```python
from build123d import *

# Parameters (mm, degrees)
SKETCH1_W                                = 75
SKETCH1_H                                = 80
BOSS_EXTRUDE1_DEPTH                      = 5
CUT_EXTRUDE1_START                       = -6
CUT_EXTRUDE1_DEPTH                       = 7
MIRROR1_START                            = -6
MIRROR1_AT_THE_SECOND_PLANE_COPY_1_DEPTH = 7
SKETCH4_R                                = 1.5875
CUT_EXTRUDE2_DEPTH                       = 6


with BuildPart() as part:
    # Sketch1 → Boss-Extrude1 (new body)
    with BuildSketch(Plane(origin=(0, 0, 0), x_dir=(0, 0, -1), z_dir=(1, 0, 0))):
        Rectangle(SKETCH1_W, SKETCH1_H)
    extrude(amount=BOSS_EXTRUDE1_DEPTH)

    # Sketch3 → Cut-Extrude1 (cut)
    with BuildSketch(Plane(origin=(5, 0, 0), x_dir=(0, 0, -1), z_dir=(1, 0, 0)).offset(CUT_EXTRUDE1_START)):
        Polygon((-37.5, 20), (-32.5, 20), (-32.5, 35), (-15, 35), (-15, 40), (-37.5, 40), align=None)
    cut_extrude1 = extrude(amount=CUT_EXTRUDE1_DEPTH, mode=Mode.SUBTRACT)

    # Mirror1: Cut-Extrude1 across plane
    add(cut_extrude1.mirror(Plane.XY), mode=Mode.SUBTRACT)

    # Mirror1 at the second plane: Cut-Extrude1 across plane
    add(cut_extrude1.mirror(Plane.ZX), mode=Mode.SUBTRACT)

    # Mirror1 at the second plane copy 1 sketc → Mirror1 at the second plane copy 1 (cut)
    with BuildSketch(Plane(origin=(5, 0, 0), x_dir=(0, 0, 1), z_dir=(1, 0, 0)).offset(MIRROR1_START)):
        Polygon((-37.5, 20), (-32.5, 20), (-32.5, 35), (-15, 35), (-15, 40), (-37.5, 40), align=None)
    extrude(amount=MIRROR1_AT_THE_SECOND_PLANE_COPY_1_DEPTH, mode=Mode.SUBTRACT)

    # Sketch4 → Cut-Extrude2 (cut, through all)
    with BuildSketch(Plane(origin=(5, 0, 0), x_dir=(0, 0, -1), z_dir=(1, 0, 0))):
        with Locations((-15, 35)):
            Circle(SKETCH4_R)
        with Locations((15, 35)):
            Circle(SKETCH4_R)
        with Locations((32.5, 20)):
            Circle(SKETCH4_R)
        with Locations((32.5, -20)):
            Circle(SKETCH4_R)
        with Locations((15, -35)):
            Circle(SKETCH4_R)
        with Locations((-15, -35)):
            Circle(SKETCH4_R)
        with Locations((-32.5, -20)):
            Circle(SKETCH4_R)
        with Locations((-32.5, 20)):
            Circle(SKETCH4_R)
    extrude(amount=-CUT_EXTRUDE2_DEPTH, mode=Mode.SUBTRACT)


solid = part.part
```
For this review, take the finished solid that the model builds, in its own axes (mm). A direction names the side the tool comes from. Round coordinates to 2 decimals unless told otherwise and drop trailing zeros. Write each loop counter-clockwise with the first axis right and the second up, starting at its lowest first coordinate (ties: lowest second). Pieces come first, ordered by that corner, then holes. Notation, with made-up numbers: (-16, -19.75) -> (10, -19.75) arc R23 cw to (10, -11.75) -> close; hole circle Ø10 at (70, -7.5). An arc over 180 degrees is marked (long way). Use one line per item in the form item = value.
Q1. Consider section B-B (y = -26). State the section outline as (x, z) points, then the cut area to 3 significant figures.
Resolved:
outline = (0, -32.5) -> (5, -32.5) -> (5, 32.5) -> (0, 32.5) -> close
area = 325 mm²
Q2. To check wall thickness, follow probe 1 along Y at (x, z) = (1.95, -25); probe 2 along Z at (x, y) = (1.8, 29.5); probe 3 along Z at (x, y) = (2.3, -34). State the ranges of each line that lie inside material, in increasing order. Write a range as from..to.
Resolved:
probe_1 = -35..35
probe_2 = -32.5..32.5
probe_3 = -32.5..-16.23, -13.77..13.77, 16.23..32.5
Q3. Clearance check with flat-ended pins moving along their axes: pin 1 Ø2.5 at (x, z) = (3.5, -36.5) entering from +Y; pin 2 Ø1.9 at (y, z) = (-35, -15) entering from +X; pin 3 Ø1 at (x, z) = (2, -26) entering from +Y; pin 4 Ø1.7 at (x, y) = (2, 39) entering from +Z. State where each tip first meets the part, or that it passes through.
Resolved:
pin_1 = 20
pin_2 = through
pin_3 = 35
pin_4 = 15
Q4. Machinability: for faces 4 (the flat face through (2, -35, 25)), 5 (the cylindrical face through (2.535, 18.915, -31.341)), 6 (the flat face through (2, 38, 15)), 7 (the flat face through (2, 35, -25)), 8 (the flat face through (2, -35, -25)), which of the approach directions +Z, -Z, +X, -X, +Y, -Y give a long, thin tool a straight path to every point of the face, cutting with its end or side? Answer none if there is none.
Resolved:
face_4 = +Z, +X, -X, -Y
face_5 = +X, -X
face_6 = +Z, +X, -X, +Y
face_7 = -Z, +X, -X, +Y
face_8 = -Z, +X, -X, -Y
Q5. Consider section A-A (x = 3). State the section outline as (y, z) points (1 decimal), then the cut area to 3 significant figures.
Resolved:
outline = (-40, -15) -> (-36.6, -15) arc R1.6 cw (long way) to (-35, -16.6) -> (-35, -32.5) -> (-21.6, -32.5) arc R1.6 cw (long way) to (-20, -34.1) -> (-20, -37.5) -> (20, -37.5) -> (20, -34.1) arc R1.6 cw (long way) to (21.6, -32.5) -> (35, -32.5) -> (35, -16.6) arc R1.6 cw (long way) to (36.6, -15) -> (40, -15) -> (40, 15) -> (36.6, 15) arc R1.6 cw (long way) to (35, 16.6) -> (35, 32.5) -> (21.6, 32.5) arc R1.6 cw (long way) to (20, 34.1) -> (20, 37.5) -> (-20, 37.5) -> (-20, 34.1) arc R1.6 cw (long way) to (-21.6, 32.5) -> (-35, 32.5) -> (-35, 16.6) arc R1.6 cw (long way) to (-36.6, 15) -> (-40, 15) -> close
area = 5,200 mm²
Q6. The part is to be moulded in two halves that separate along Z. For faces 1 (the flat face through (2, 0, 37.5)), 2 (the flat face through (2, 28, -32.5)), 3 (the cylindrical face through (2.535, -33.841, -13.915)), say which applies: released by +Z, released by -Z, zero draft, split by the parting line, or undercut.
Resolved:
face_1 = released by +Z
face_2 = released by -Z
face_3 = undercut
